```python
from build123d import *

# Parameters (mm, degrees)
F0_W     = 46
F0_H     = 32
F1_DEPTH = 2.5
F2_R     = 6
F3_DEPTH = 0.5
F4_R     = 1


with BuildPart() as f1:
    # F0 (on Top) → F1 (new body)
    with BuildSketch(Plane.XY):
        Rectangle(F0_W, F0_H)
    extrude(amount=F1_DEPTH)

    # F2 (on face) → F3 (join)
    with BuildSketch(Plane.XY.offset(2.5)):
        with Locations((-15, 8)):
            Circle(F2_R)
        with Locations((15, 8)):
            Circle(F2_R)
        with Locations((-15, -8)):
            Circle(F2_R)
        with Locations((15, -8)):
            Circle(F2_R)
    extrude(amount=F3_DEPTH)

    # F4
    f4_edges = [f1.edges().sort_by_distance(p)[0] for p in [
        (23, -16, 1.25),
        (-23, -16, 1.25),
        (23, 16, 1.25),
        (-23, 16, 1.25),
    ]]
    fillet(f4_edges, radius=F4_R)


solid = f1.part
```
Source: CAD feature listing. Evaluate the final solid. Frame: model axes, mm. A direction names the side the tool comes from. Give positions to 0.01 mm unless a question says otherwise; leave off trailing zeros. Write each loop counter-clockwise with the first axis right and the second up, starting at its lowest first coordinate (ties: lowest second). Pieces come first, ordered by that corner, then holes. Notation, with made-up numbers: (-18.75, 80) - (25.25, 80) arc R12 ccw to (25.25, 101) - close; hole circle Ø11 at (27, -4.5). An arc over 180 degrees is marked (long way). One line per item, written item: value. Start each with the question number.
Q1. Draft query along X for faces 1 (the face through (-9.277, -6.198, 2.746)), 2 (the face through (-15, 8, 3)), 3 (the face through (-23, 0, 1)). Return one class per face: +X half, -X half, draft (parallel to the pull), parting line (faces both ways), or undercut.
Q2. Section query B-B, the plane x = 15. Return the cut outline in (y, z).
Q3. First-contact query: pin 1 Ø1.5 at (x, y) = (-4, -0.5) entering from +Z; pin 2 Ø2 at (x, y) = (-3, -2) entering from -Z. Flat tips, straight axial feed; report the tip coordinate or a pass-through.
Q4. Set-up query: faces 4 (the face through (-9.46, 5.7, 2.75)), 5 (the face through (0, 16, 1)). Return all of +Z, -Z, +X, -X, +Y, -Y with unobstructed straight access to the full face (end or side cutting, diameter ignored); none if empty.
Q5. Section query A-A, the plane y = 8. Return the cut outline in (x, z).
Q6. Material intervals for probe 1 along Z at (x, y) = (13, 1); probe 2 along X at (y, z) = (-3, 2.75); probe 3 along X at (y, z) = (5.5, 2.8), sorted ascending. Write a range as from..to.
Q7. Section query C-C, the plane x = -3.5. Return the cut outline in (y, z).
Answer:
1. face 1: undercut
1. face 2: draft
1. face 3: -X half
2. outline: (-16, 0) - (16, 0) - (16, 2.5) - (14, 2.5) - (14, 3) - (2, 3) - (2, 2.5) - (-2, 2.5) - (-2, 3) - (-14, 3) - (-14, 2.5) - (-16, 2.5) - close
3. pin 1: stops at z = 2.5
3. pin 2: stops at z = 0
4. face 4: +Z
4. face 5: +Z, -Z, +X, -X, +Y
5. outline: (-23, 0) - (23, 0) - (23, 2.5) - (21, 2.5) - (21, 3) - (9, 3) - (9, 2.5) - (-9, 2.5) - (-9, 3) - (-21, 3) - (-21, 2.5) - (-23, 2.5) - close
6. probe 1: z = 0..2.5
6. probe 2: x = -18.32..-11.68, 11.68..18.32
6. probe 3: x = -20.45..-9.55, 9.55..20.45
7. outline: (-16, 0) - (16, 0) - (16, 2.5) - (-16, 2.5) - close
